Source: CAD feature listing. Evaluate the final solid. Frame: model axes, mm. A direction names the side the tool comes from. Give positions to 0.01 mm unless a question says otherwise; leave off trailing zeros. Loops run counter-clockwise (first coordinate to the right, second up) from the corner with the lowest first, then second, coordinate; pieces in that order, holes last. Notation, with made-up numbers: (52.25, -3) -> (91.25, -3) arc R8 cw to (91.25, 1) -> close; hole circle Ø11 at (-24.5, 69). An arc over 180 degrees is marked (long way). Return JSON: item names as keys, results as strings. Group by question number.
```python
from build123d import *

# Parameters (mm, degrees)
SKETCH_1_R          = 1.5
EXTRUDE_1_DEPTH     = 2
FILLET_2_R          = 5
FILLET_3_R          = 5
SKETCH_7_R          = 6
CUT_EXTRUDE_4_DEPTH = 10
FILLET_5_R          = 5
SKETCH_10_W         = 10
SKETCH_10_H         = 2
EXTRUDE_4_DEPTH     = 10


with BuildPart() as part:
    # 草图1 → 凸台-拉伸1 (new body)
    with BuildSketch(Plane(origin=(0, 0, 0), x_dir=(1, 0, 0), z_dir=(0, 1, 0))):
        with BuildLine():
            Line((17.196152423, -13), (52, -13))
            Line((52, -13), (52, -5))
            Line((52, -5), (-15, -5))
            Line((-15, -5), (-15, 5))
            Line((-15, 5), (-25, 5))
            Line((-25, 5), (-25, -13))
            Line((-25, -13), (6.803847577, -13))
            ThreePointArc((6.803847577, -13), (12, -16), (17.196152423, -13))
        make_face()
        with Locations(Location((-20, 0, 0), (0, 0, 270))):
            Circle(SKETCH_1_R, mode=Mode.SUBTRACT)
    extrude(amount=EXTRUDE_1_DEPTH)

    # 圆角2
    fillet_2_edges = [part.edges().sort_by_distance(p)[0] for p in [
        (-25, 1, -5),
    ]]
    fillet(fillet_2_edges, radius=FILLET_2_R)

    # 圆角3
    fillet_3_edges = [part.edges().sort_by_distance(p)[0] for p in [
        (-25, 1, 13),
    ]]
    fillet(fillet_3_edges, radius=FILLET_3_R)

    # 草图7 → 切除-拉伸4 (cut)
    with BuildSketch(Plane(origin=(0, 2, 0), x_dir=(1, 0, 0), z_dir=(0, 1, 0))):
        with Locations((12, -2)):
            Circle(SKETCH_7_R)
    extrude(amount=-CUT_EXTRUDE_4_DEPTH, mode=Mode.SUBTRACT)

    # 圆角5
    fillet_5_edges = [part.edges().sort_by_distance(p)[0] for p in [
        (17.196152423, 1, 13),
        (6.803847577, 1, 13),
        (6.803847577, 1, 5),
        (17.196152423, 1, 5),
    ]]
    fillet(fillet_5_edges, radius=FILLET_5_R)

    # 草图10 → 凸台-拉伸4 (add)
    with BuildSketch(Plane(origin=(-15, 0, 0), x_dir=(0, 0, -1), z_dir=(1, 0, 0))):
        with Locations((0, 1)):
            Rectangle(SKETCH_10_W, SKETCH_10_H)
    extrude(amount=EXTRUDE_4_DEPTH)


solid = part.part
```
1) Cut plane C-C on x = -10. Return loops of the section in (y, z).
2) Reachability of faces 1 (the face through (36, 1, 13)), 2 (the face through (17.679, 1.014, 5.363)), 3 (the face through (-8, 1, 13)), 4 (the face through (36, 1, 5)) from +Z, -Z, +X, -X, +Y, -Y: full face, straight path, thin tool, end or side. Return the list, or none.
3) Cut plane B-B on x = 34.5. Return loops of the section in (y, z), then the cut area to 3 significant figures.
4) Cut plane A-A on y = 1.4. Return loops of the section in (x, z), then the cut area to 3 significant figures.
5) Material intervals for line 1 (X direction, y = 1.15, z = 0); line 2 (Z direction, x = 38, y = 0.25); line 3 (Z direction, x = -10.5, y = 1.5), sorted ascending.
6) Contact query for flat-ended pins moving along their axis: P1, Ø2.5, axis at x = -20, z = 0, coming from the -Y side; P2, Ø1, axis at x = 0, y = 1.5, coming from the +Z side; P3, Ø0.6, axis at y = 1, z = 0, coming from the +X side; P4, Ø0.6, axis at x = 35.5, y = 1.5, coming from the -Z side. Output: stop coordinate, or through.
7) Mould query, pull axis Z, two halves, no side actions, for faces 5 (the face through (4, 0, 8)), 6 (the face through (6.272, 1.014, 5.344)), 7 (the face through (-18.735, 0.986, 0.806)), 8 (the face through (6.321, 1.014, 13.363)). Classes: released by +Z, released by -Z, zero draft, split by the parting line, or undercut.
Calculated:
{
 "1": {"outline": "(0, -5) -> (2, -5) -> (2, 13) -> (0, 13) -> close"},
 "2": {"face 1": "+Z, +X, +Y, -Y", "face 2": "-Z, +Y, -Y", "face 3": "+Z, -X, +Y, -Y", "face 4": "-Z, +X, +Y, -Y"},
 "3": {"outline": "(0, 5) -> (2, 5) -> (2, 13) -> (0, 13) -> close", "area": "16.0 mm2"},
 "4": {"outline": "(-25, 0) arc R5 ccw to (-20, -5) -> (-5, -5) -> (-5, 5) -> (4.45, 5) arc R5 ccw to (7.88, 6.36) arc R6 cw to (16.12, 6.36) arc R5 ccw to (19.55, 5) -> (52, 5) -> (52, 13) -> (19.55, 13) arc R5 cw to (16.12, 14.36) arc R6 ccw to (7.88, 14.36) arc R5 cw to (4.45, 13) -> (-20, 13) arc R5 ccw to (-25, 8) -> close; hole circle Ø3 at (-20, 0)", "area": "798 mm2"},
 "5": {"line 1": "-25 to -21.5, -18.5 to -5", "line 2": "5 to 13", "line 3": "-5 to 13"},
 "6": {"P1": "through", "P2": "z = 13", "P3": "x = -5", "P4": "z = 5"},
 "7": {"face 5": "zero draft", "face 6": "released by -Z", "face 7": "undercut", "face 8": "released by +Z"}
}
